Here's how the part is built. I have some questions about the finished solid (model axes, mm). A direction names the side the tool comes from. Round coordinates to 2 decimals unless told otherwise and drop trailing zeros. Write each loop counter-clockwise with the first axis right and the second up, starting at its lowest first coordinate (ties: lowest second). Pieces come first, ordered by that corner, then holes. Notation, with made-up numbers: (-25.75, 17) -> (22.25, 17) arc R16 ccw to (22.25, 45) -> close; hole circle Ø2 at (-6.5, -5.5). An arc over 180 degrees is marked (long way). Answer as CSV lines item,"result".
from build123d import *

# Parameters (mm, degrees)
SKETCH_1_W          = 40
SKETCH_1_H          = 4
EXTRUDE_1_DEPTH     = 40
SKETCH_3_W          = 40
SKETCH_3_H          = 30
CUT_EXTRUDE_1_DEPTH = 2
SKETCH_4_R          = 1
CUT_EXTRUDE_2_DEPTH = 4
SKETCH_6_R          = 1
CUT_EXTRUDE_3_DEPTH = 4
FILLET_4_R          = 10
FILLET_5_R          = 10
FILLET_6_R          = 2
FILLET_7_R          = 2
FILLET_8_R          = 2


with BuildPart() as part:
    # ｽｹｯﾁ1 → ﾎﾞｽ - 押し出し1 (new body)
    with BuildSketch(Plane.XY):
        with Locations((20, 2)):
            Rectangle(SKETCH_1_W, SKETCH_1_H)
    extrude(amount=EXTRUDE_1_DEPTH)

    # ｽｹｯﾁ3 → ｶｯﾄ - 押し出し1 (cut)
    with BuildSketch(Plane.XZ):
        with Locations((20, 25)):
            Rectangle(SKETCH_3_W, SKETCH_3_H)
    extrude(amount=-CUT_EXTRUDE_1_DEPTH, mode=Mode.SUBTRACT)

    # ｽｹｯﾁ4 → ｶｯﾄ - 押し出し2 (cut)
    with BuildSketch(Plane(origin=(0, 4, 0), x_dir=(1, 0, 0), z_dir=(0, 1, 0))):
        with Locations(Location((35.5, -20, 0), (0, 0, 270))):
            Circle(SKETCH_4_R)
    extrude(amount=-CUT_EXTRUDE_2_DEPTH, mode=Mode.SUBTRACT)

    # ｽｹｯﾁ6 → ｶｯﾄ - 押し出し3 (cut)
    with BuildSketch(Plane(origin=(0, 4, 0), x_dir=(1, 0, 0), z_dir=(0, 1, 0))):
        with Locations(Location((5, -20, 0), (0, 0, 270))):
            Circle(SKETCH_6_R)
    extrude(amount=-CUT_EXTRUDE_3_DEPTH, mode=Mode.SUBTRACT)

    # ﾌｨﾚｯﾄ4
    fillet_4_edges = [part.edges().sort_by_distance(p)[0] for p in [
        (40, 3, 40),
    ]]
    fillet(fillet_4_edges, radius=FILLET_4_R)

    # ﾌｨﾚｯﾄ5
    fillet_5_edges = [part.edges().sort_by_distance(p)[0] for p in [
        (0, 3, 40),
    ]]
    fillet(fillet_5_edges, radius=FILLET_5_R)

    # ﾌｨﾚｯﾄ6
    fillet_6_edges = [part.edges().sort_by_distance(p)[0] for p in [
        (0, 4, 15),
        (2.928932188, 4, 37.071067812),
        (20, 4, 40),
        (37.071067812, 4, 37.071067812),
        (40, 4, 15),
    ]]
    fillet(fillet_6_edges, radius=FILLET_6_R - 0.0001)  # a hair under: the kernel refuses the full size

    # ﾌｨﾚｯﾄ7
    fillet_7_edges = [part.edges().sort_by_distance(p)[0] for p in [
        (40, 0, 5),
    ]]
    fillet(fillet_7_edges, radius=FILLET_7_R)

    # ﾌｨﾚｯﾄ8
    fillet_8_edges = [part.edges().sort_by_distance(p)[0] for p in [
        (0, 0, 5),
    ]]
    fillet(fillet_8_edges, radius=FILLET_8_R)


solid = part.part
Item 1: If we mould it in two halves opening along Z, with no side actions, what happens to faces 3 (the cylindrical face through (36.49, 3.01, 19.87)), 4 (the cylindrical face through (0.6, 0.57, 5.07)), 5 (the cylindrical face through (5.676, 3.014, 19.263)), 6 (the flat face through (20, 1, 10))? For each: pulls with the +Z half, pulls with the -Z half, needs draft (parallel to the pull), parting line crosses it, or undercut.
Results found:
face 3,"undercut"
face 4,"needs draft"
face 5,"undercut"
face 6,"pulls with the +Z half"
Item 2: Suppose I cut it at C-C, the plane y = 3.3. List the corners of the cut face in (x, z) for me.
Results found:
outline,"(0.48, 0) -> (39.52, 0) -> (39.52, 30) arc R9.52 ccw to (30, 39.52) -> (10, 39.52) arc R9.52 ccw to (0.48, 30) -> close; hole circle Ø2 at (5, 20); hole circle Ø2 at (35.5, 20)"
Item 3: Suppose I cut it at A-A, the plane z = 20. State how many separate pieces and enclosed holes the cut face has, then the cut area to 3 significant figures.
Results found:
separate pieces,"3"
enclosed holes,"0"
area,"70.3 mm²"
Item 4: I need wall thicknesses on L1, parallel to X at y = 3.6, z = 20; L2, parallel to X at y = 2.9, z = 20; L3, parallel to Y at x = 35.5, z = 33. Which ranges of each line are inside material? Lowest first, please.
Results found:
L1,"x = 0.8 to 4, 6 to 34.5, 36.5 to 39.2"
L2,"x = 0.21 to 4, 6 to 34.5, 36.5 to 39.79"
L3,"y = 2 to 4"
Item 5: For faces 1 (the cylindrical face through (20.14, 3.43, 39.4)), 2 (the flat face through (20, 2, 25)), which set-ups out of +Z, -Z, +X, -X, +Y, -Y let a thin tool reach every point of the face, with its end or its side?
Results found:
face 1,"+Z, +X, -X, +Y"
face 2,"+Z, +X, -X, -Y"
Item 6: Will these pins go through, and if not, where does the flat tip stop? pin 1 (24 mm diameter, centred on x = 17, z = 23.5, fed in from -Y); pin 2 (0.6 mm diameter, centred on x = 16, y = 1, fed in from +Z); pin 3 (1.5 mm diameter, centred on y = 1, z = 10, fed in from -X).
Results found:
pin 1,"stops at y = 2"
pin 2,"stops at z = 10"
pin 3,"stops at x = 0.02"
